from build123d import *

# Parameters (mm, degrees)
BOSS_EXTRUDE1_DEPTH                                 = 12.7
CBORE_FOR_M6_HEX_SOCKET_HEAD_CAP_SCREW1_D           = 6.6
CBORE_FOR_M6_HEX_SOCKET_HEAD_CAP_SCREW1_CBORE_D     = 11
CBORE_FOR_M6_HEX_SOCKET_HEAD_CAP_SCREW1_CBORE_DEPTH = 7
CUT_EXTRUDE1_DEPTH                                  = 58.938313101


with BuildPart() as part:
    # Sketch1 → Boss-Extrude1 (new, symmetric)
    with BuildSketch(Plane(origin=(0, 0, 0), x_dir=(0, 0, -1), z_dir=(1, 0, 0))):
        Polygon((-41.275, 0), (41.275, 0), (41.275, 25.4), (23.828518386, 31.75), (-23.828518386, 31.75), (-41.275, 25.4), align=None)
    extrude(amount=BOSS_EXTRUDE1_DEPTH, both=True)

    # CBORE for M6 Hex Socket Head Cap Screw1 (through all)
    with Locations(Plane(origin=(12.7, 13.34258249, -21.373421522), x_dir=(0, 1, 0), z_dir=(1, 0, 0))):
        with Locations((-0.64258249, 33.873421522), (-0.64258249, 8.873421522)):
            CounterBoreHole(CBORE_FOR_M6_HEX_SOCKET_HEAD_CAP_SCREW1_D / 2, CBORE_FOR_M6_HEX_SOCKET_HEAD_CAP_SCREW1_CBORE_D / 2, CBORE_FOR_M6_HEX_SOCKET_HEAD_CAP_SCREW1_CBORE_DEPTH)

    # Sketch5 → Cut-Extrude1 (cut, through all)
    with BuildSketch(Plane(origin=(12.7, 0, 0), x_dir=(0, 0, -1), z_dir=(1, 0, 0))):
        with BuildLine():
            Line((15.2, -15), (15.2, -6.7))
            ThreePointArc((15.2, -6.7), (11.480256121, 2.280256121), (2.5, 6))
            Line((2.5, 6), (-2.5, 6))
            ThreePointArc((-2.5, 6), (-11.480256121, 2.280256121), (-15.2, -6.7))
            Line((-15.2, -6.7), (-15.2, -15))
            Line((-15.2, -15), (15.2, -15))
        make_face()
    extrude(amount=-CUT_EXTRUDE1_DEPTH, mode=Mode.SUBTRACT)


solid = part.part
Check sheet for the modelled part. Datum: model origin and axes. Units: mm. A direction names the side the tool comes from. Give positions to 0.01 mm unless a question says otherwise; leave off trailing zeros. Write each loop counter-clockwise with the first axis right and the second up, starting at its lowest first coordinate (ties: lowest second). Pieces come first, ordered by that corner, then holes. Notation, with made-up numbers: M -2.75,-7.75 L 20.25,-7.75 A23 ccw 20.25,26.25 Z; hole C 80,73.25 d7. An arc over 180 degrees is marked long. Use one line per item in the form item = value.
(1) Section check C-C on z = -14.5. Record the boundary of the cut face in (x, y).
Answer block:
outline = M -12.7,0 L 12.7,0 L 12.7,7.58 L 5.7,7.58 L 5.7,10.08 L -12.7,10.08 Z; M -12.7,15.32 L 5.7,15.32 L 5.7,17.82 L 12.7,17.82 L 12.7,31.75 L -12.7,31.75 Z
(2) Draft check along Z on faces 1 (the flat face through (12.7, 16, 1)), 2 (the cylindrical face through (-3.63, 13.42, 9.28)), 3 (the flat face through (0.18, 28.53, -32.67)). Enter one of: pulls with the +Z half, pulls with the -Z half, needs draft (parallel to the pull), parting line crosses it, or undercut.
Answer block:
face_1 = needs draft
face_2 = undercut
face_3 = pulls with the -Z half
(3) Section check B-B on x = 8.25. Record the boundary of the cut face in (y, z) (3 decimals), plus the area to 3 significant figures.
Answer block:
outline = M 0,-41.275 L 25.4,-41.275 L 31.75,-23.829 L 31.75,23.829 L 25.4,41.275 L 0,41.275 L 0,13.289 A12.7 cw 6,2.5 L 6,-2.5 A12.7 cw 0,-13.289 Z; hole C 12.7,-12.5 d11; hole C 12.7,12.5 d11
area = 2,200 mm2
(4) Tool access check on faces 4 (the cylindrical face through (9.2, 8.3, -15.8)), 5 (the cylindrical face through (0.178, 4.355, -8.751)), 6 (the flat face through (0.18, 28.62, 32.43)). Record the directions out of +Z, -Z, +X, -X, +Y, -Y that give a thin tool (end or side, any length) a straight path to the whole face; none if there is none.
Answer block:
face_4 = +X
face_5 = +X, -X, -Y
face_6 = +Z, +X, -X, +Y
(5) Material ranges on line 1 along Z through (x, y) = (10.75, 12.7) (3 decimals); line 2 along Z through (x, y) = (-6, 12.7) (3 decimals); line 3 along X through (y, z) = (13.5, 17), recorded low to high.
Answer block:
line_1 = -41.275 to -18, -7 to 7, 18 to 41.275
line_2 = -41.275 to -15.8, -9.2 to 9.2, 15.8 to 41.275
line_3 = -12.7 to 5.7
(6) Section check A-A on y = 12.7. Record the boundary of the cut face in (x, z) (3 decimals), plus the area to 3 significant figures.
Answer block:
outline = M -12.7,-41.275 L 12.7,-41.275 L 12.7,-18 L 5.7,-18 L 5.7,-15.8 L -12.7,-15.8 Z; M -12.7,-9.2 L 5.7,-9.2 L 5.7,-7 L 12.7,-7 L 12.7,7 L 5.7,7 L 5.7,9.2 L -12.7,9.2 Z; M -12.7,15.8 L 5.7,15.8 L 5.7,18 L 12.7,18 L 12.7,41.275 L -12.7,41.275 Z
area = 1,700 mm2
(7) Section check D-D on y = 3. Record the boundary of the cut face in (x, z) (3 decimals).
Answer block:
outline = M -12.7,-41.275 L 12.7,-41.275 L 12.7,-10.698 L -12.7,-10.698 Z; M -12.7,10.698 L 12.7,10.698 L 12.7,41.275 L -12.7,41.275 Z
(8) Depth check by flat-ended pin: P1, Ø10, axis at y = 12.7, z = 12.5, coming from the +X side; P2, Ø1, axis at x = 2, z = -27.5, coming from the +Y side; P3, Ø4, axis at x = -1.5, z = 0, coming from the -Y side. Enter the tip coordinate at first touch or a pass-through.
Answer block:
P1 = 5.7
P2 = 30.6
P3 = 6
